Geometry check sheet. Reference: drawing and pictorial views, mm from the part's lowest x, y, z. A direction names the side the tool comes from. Coordinates: 2 decimals unless noted, no trailing zeros. Loops run counter-clockwise (first coordinate to the right, second up) from the corner with the lowest first, then second, coordinate; pieces in that order, holes last. Notation, with made-up numbers: (66.25, 3.25) -> (118.25, 3.25) arc R22 cw to (118.25, 21.25) -> close; hole circle Ø4 at (1.5, 0.25). An arc over 180 degrees is marked (long way). Answer as a JSON object with one key per item and string values.
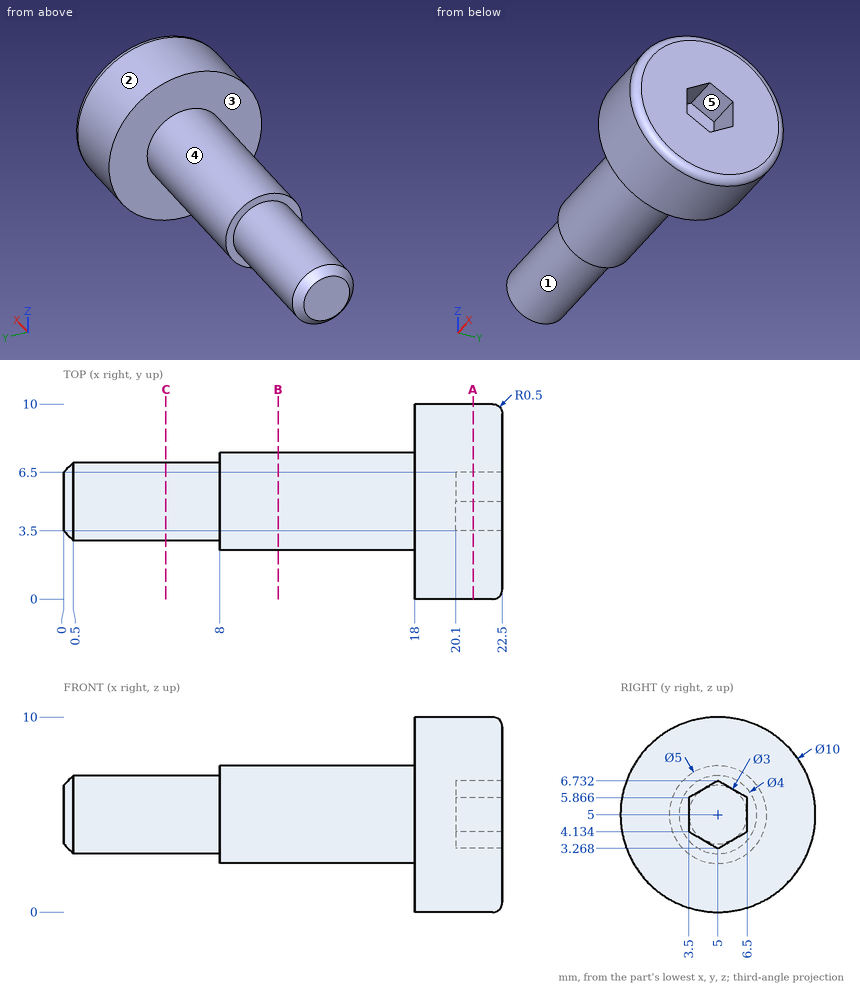
1. Depth check by flat-ended pin: P1, Ø1.5, axis at x = 14.5, z = 7.5, coming from the -Y side; P2, Ø3.5, axis at y = 4.5, z = 5, coming from the +X side; P3, Ø3, axis at x = 6.5, z = 8, coming from the +Y side; P4, Ø0.5, axis at x = 21.5, z = 5.5, coming from the +Y side. Enter the tip coordinate at first touch or a pass-through.
Evaluation:
{"P1": "stops at y = 3.21", "P2": "stops at x = 22.5", "P3": "stops at y = 6.32", "P4": "stops at y = 9.99"}
2. Section check A-A, the plane x = 21. Record the boundary of the cut face in (y, z).
Evaluation:
{"outline": "circle Ø10 at (5, 5); hole (3.5, 4.13) -> (5, 3.27) -> (6.5, 4.13) -> (6.5, 5.87) -> (5, 6.73) -> (3.5, 5.87) -> close"}
3. Mould release check, pull along Y, two halves, no side actions. Record for the marked faces 3, 4 and 5: released by +Y, released by -Y, zero draft, split by the parting line, or undercut.
Evaluation:
{"face 3": "zero draft", "face 4": "split by the parting line", "face 5": "undercut"}
4. Section check C-C, the plane x = 5.25. Record the boundary of the cut face in (y, z), then the cut area to 3 significant figures.
Evaluation:
{"outline": "circle Ø4 at (5, 5)", "area": "12.6 mm^2"}
5. Tool access check on the marked faces 1 and 2. Record the directions out of +Z, -Z, +X, -X, +Y, -Y that give a thin tool (end or side, any length) a straight path to the whole face; none if there is none.
Evaluation:
{"face 1": "-X", "face 2": "+X, -X"}
6. Thickness scan on probe 1 along X at (y, z) = (7.5, 6.75); probe 2 along Z at (x, y) = (1.5, 6); probe 3 along Y at (x, z) = (9.75, 6.5). Record the ranges inside material, lowest first. Write a range as from..to.
Evaluation:
{"probe 1": "x = 18..22.5", "probe 2": "z = 3.27..6.73", "probe 3": "y = 3..7"}
7. Section check B-B, the plane x = 11. Record the boundary of the cut face in (y, z), then the cut area to 3 significant figures.
Evaluation:
{"outline": "circle Ø5 at (5, 5)", "area": "19.6 mm^2"}
